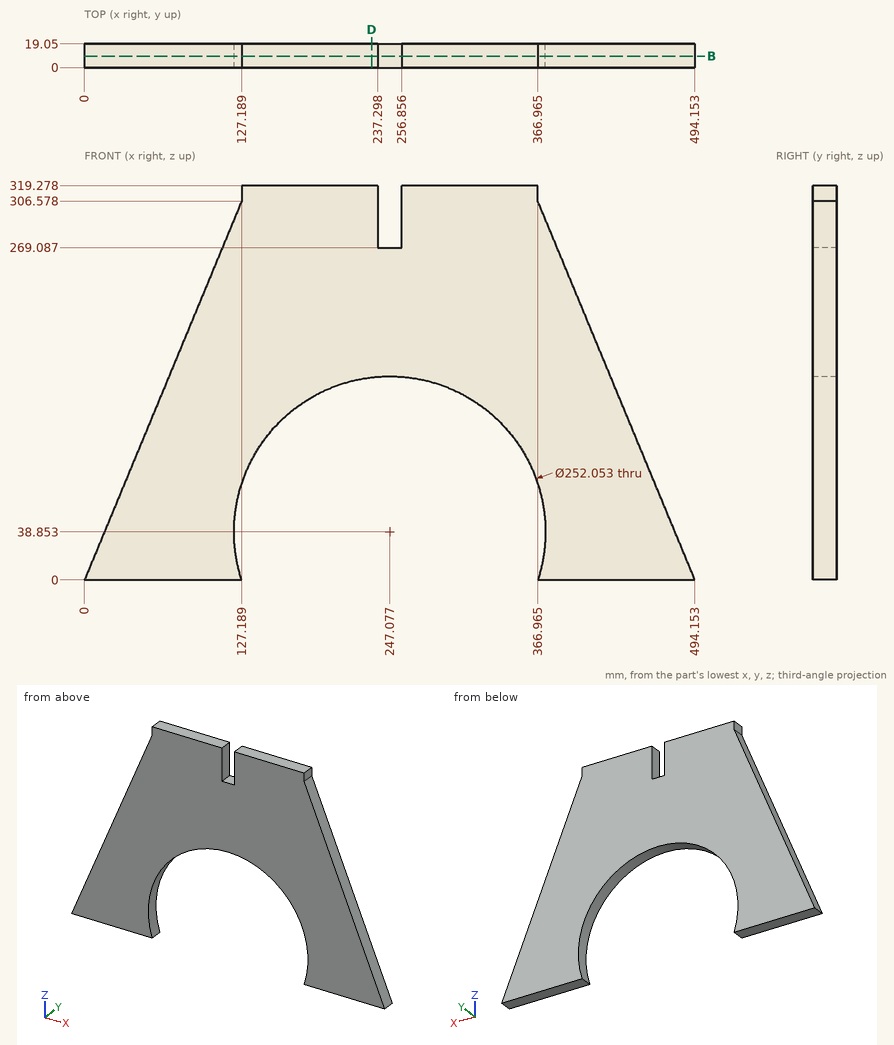
Print and shaded views of the part. All mm, measured from the part's lowest x, y and z. Give positions to 0.01 mm unless a question says otherwise; leave off trailing zeros. Order: outer loops, then holes, each group sorted by start corner. A loop starts at its lowest first (then second) coordinate and runs counter-clockwise, first axis right, second up. Notation, with made-up numbers: (46, 50) - (51, 50) arc R31 ccw to (51, 88) - close; hole circle Ø4 at (37, -0.75). An arc over 180 degrees is marked (long way). Use a Markdown table: item, result.
1) Saw through at D-D on x = 232.5. List the corners of the cut face in (y, z), plus the area to 3 significant figures.
Checked values:
| item | result |
|---|---|
| outline | (0, 164.03) - (19.05, 164.03) - (19.05, 319.28) - (0, 319.28) - close |
| area | 2,960 mm² |
2) Probe L1, parallel to X at y = 6.5, z = 291.5 (1 decimal); L2, parallel to X at y = 12.75, z = 132 (1 decimal); L3, parallel to Z at x = 42.5, y = 2.75 (1 decimal). List the from-to ranges inside material, lowest first. Write a range as from..to.
Checked values:
| item | result |
|---|---|
| L1 | 120.9..237.3, 256.9..373.2 |
| L2 | 54.8..162.2, 332..439.4 |
| L3 | 0..102.4 |
3) Flat gauge pins, fed straight in: P1, Ø5.5, axis at x = 247.5, y = 9, coming from the +Z side; P2, Ø3, axis at x = 316, y = 4, coming from the -Z side; P3, Ø6.5, axis at y = 12, z = 316, coming from the +X side (1 decimal). Where does each tip first touch, or does it go through?
Checked values:
| item | result |
|---|---|
| P1 | z = 269.09 |
| P2 | z = 143.37 |
| P3 | x = 367 |
4) Saw through at B-B on y = 9.25. List the corners of the cut face in (x, z) (1 decimal).
Checked values:
| item | result |
|---|---|
| outline | (0, 0) - (127.2, 0) arc R126 cw (long way) to (367, 0) - (494.2, 0) - (367, 306.6) - (367, 319.3) - (256.9, 319.3) - (256.9, 269.1) - (237.3, 269.1) - (237.3, 319.3) - (127.2, 319.3) - (127.2, 306.6) - close |
